Read the model definition and answer for the solid it produces. Units are mm, in the model's axes. A direction names the side the tool comes from. Give positions to 0.01 mm unless a question says otherwise; leave off trailing zeros. Loops run counter-clockwise (first coordinate to the right, second up) from the corner with the lowest first, then second, coordinate; pieces in that order, holes last. Notation, with made-up numbers: (-25, 34.5) - (26, 34.5) arc R28 ccw to (26, 60.5) - close; hole circle Ø5 at (2.5, 16). An arc over 180 degrees is marked (long way). Use a Markdown table: item, result. Add a question column.
Item 1: Each of these flat-tipped pins is pushed along its axis until it touches: P1, Ø4, axis at x = 12, y = 29.5, coming from the +Z side; P2, Ø11, axis at x = 16.5, y = -29.5, coming from the -Z side; P3, Ø1, axis at x = 5.5, y = -3, coming from the +Z side; P4, Ø12.5, axis at x = 17, z = 15, coming from the +Y side. Where does it stop, or does it pass through?
Item 2: Consider probe 1 along Y at (x, z) = (2.25, 13.5); probe 2 along Z at (x, y) = (8.5, 32.5); probe 3 along X at (y, z) = (31, 13). Determine where each line is inside the solid, lowest interval first. Write a range as [from, to].
Item 3: A cutting plane is placed at B-B (x = 16.75). Determine the outline of the cut face in (y, z).
Item 4: A cutting plane is placed at C-C (z = 21.5). Determine the outline of the cut face in (x, y).
Item 5: Which of the six approach directions +Z, -Z, +X, -X, +Y, -Y give full straight-line access (tool end or side, diameter ignored) to faces 1 (the face through (13, 30, 27.562)), 2 (the face through (4, 23.142, 14)), 3 (the face through (6.161, 30, 14))?
Item 6: For a pull along Z with two mould halves and no side action, classify faces 4 (the face through (13, 30, 7.712)), 5 (the face through (13, -28, -11.28)), 6 (the face through (13, -28, 20.547)), 7 (the face through (13, 36.632, 3)) as +Z half, -Z half, draft (parallel to the pull), parting line (faces both ways), or undercut.
Item 7: A cutting plane is placed at D-D (y = 30). Determine the outline of the cut face in (x, z).
Item 8: A cutting plane is placed at A-A (z = 11). Determine the outline of the cut face in (x, y), plus the area to 3 significant figures.
from build123d import *

# Parameters (mm, degrees)
F1_DEPTH = 25.4
F2_DEPTH = 25.4
F3_W     = 12.7
F3_H     = 12.7
F4_DEPTH = 50.8
F5_W     = 12.7
F5_H     = 12.7
F6_DEPTH = 50.8


with BuildPart() as f1:
    # F0 (on Right) → F1 (new body)
    with BuildSketch(Plane.YZ):
        Polygon((-21.049142, 27.794171), (-34.771789, 27.794171), (-34.771789, -11.280479), (-21.049142, -11.280479), (-21.049142, -11.513066), (23.142429, -11.513066), (36.632486, -11.513066), (36.632486, 27.561583), (23.142429, 27.561583), (23.142429, 0), (-21.049142, 0), align=None)
    extrude(amount=F1_DEPTH)

    # F0 (on Right) → F2 (join)
    with BuildSketch(Plane.YZ):
        Polygon((-21.049142, 27.794171), (-34.771789, 27.794171), (-34.771789, -11.280479), (-21.049142, -11.280479), (-21.049142, -11.513066), (23.142429, -11.513066), (36.632486, -11.513066), (36.632486, 27.561583), (23.142429, 27.561583), (23.142429, 0), (-21.049142, 0), align=None)
    extrude(amount=F2_DEPTH)

    # F3 (on face) → F4 (cut)
    with BuildSketch(Plane.XZ.offset(34.771789)):
        with Locations((12.642618, 14.197407)):
            Rectangle(F3_W, F3_H)
    extrude(amount=-F4_DEPTH, mode=Mode.SUBTRACT)

    # F5 (on face) → F6 (cut)
    with BuildSketch(Plane(origin=(0, 36.632486, 0), x_dir=(-1, 0, 0), z_dir=(0, 1, 0))):
        with Locations((-12.511186, 14.061676)):
            Rectangle(F5_W, F5_H)
    extrude(amount=-F6_DEPTH, mode=Mode.SUBTRACT)


solid = f1.part
Geometry says:
| question | item | result |
|---|---|---|
| 1 | P1 | z = 27.56 |
| 1 | P2 | z = -11.28 |
| 1 | P3 | z = 0 |
| 1 | P4 | y = 36.63 |
| 2 | probe 1 | [-34.77, -21.05], [23.14, 36.63] |
| 2 | probe 2 | [-11.51, 7.71], [20.41, 27.56] |
| 2 | probe 3 | [0, 6.16], [18.86, 25.4] |
| 3 | outline | (-34.77, -11.28) - (-21.05, -11.28) - (-21.05, -11.51) - (36.63, -11.51) - (36.63, 7.71) - (23.14, 7.71) - (23.14, 0) - (-21.05, 0) - (-21.05, 7.85) - (-34.77, 7.85) - close; (-34.77, 20.55) - (-21.05, 20.55) - (-21.05, 27.79) - (-34.77, 27.79) - close; (23.14, 20.41) - (36.63, 20.41) - (36.63, 27.56) - (23.14, 27.56) - close |
| 4 | outline | (0, -34.77) - (25.4, -34.77) - (25.4, -21.05) - (0, -21.05) - close; (0, 23.14) - (25.4, 23.14) - (25.4, 36.63) - (0, 36.63) - close |
| 5 | face 1 | +Z, +X, -X, +Y |
| 5 | face 2 | +Z, +X, -X |
| 5 | face 3 | +Y |
| 6 | face 4 | undercut |
| 6 | face 5 | -Z half |
| 6 | face 6 | undercut |
| 6 | face 7 | draft |
| 7 | outline | (0, -11.51) - (25.4, -11.51) - (25.4, 27.56) - (0, 27.56) - close; hole (6.16, 7.71) - (18.86, 7.71) - (18.86, 20.41) - (6.16, 20.41) - close |
| 8 | outline | (0, -34.77) - (6.29, -34.77) - (6.29, -21.05) - (0, -21.05) - close; (0, 23.14) - (6.16, 23.14) - (6.16, 36.63) - (0, 36.63) - close; (18.86, 23.14) - (25.4, 23.14) - (25.4, 36.63) - (18.86, 36.63) - close; (18.99, -34.77) - (25.4, -34.77) - (25.4, -21.05) - (18.99, -21.05) - close |
| 8 | area | 346 mm² |
